```python
from build123d import *

# Parameters (mm, degrees)
BOLT_CIRCLE_R                                     = 14.2748
BOLT_CIRCLE_R_2                                   = 6.35
BASE_DEPTH                                        = 12.7
STRUCTURE_TUBE_CONNECTION_COUNTERBORE_D           = 6.7564
STRUCTURE_TUBE_CONNECTION_COUNTERBORE_CBORE_D     = 11.1125
STRUCTURE_TUBE_CONNECTION_COUNTERBORE_CBORE_DEPTH = 6.35
STRUCTURE_TUBE_CONNECTION_COUNTERBORE_PA_COUNT    = 4
SPINDLE_CONNECTION_COUNTERBORE_D                  = 6.7564
SPINDLE_CONNECTION_COUNTERBORE_CBORE_D            = 11.1125
SPINDLE_CONNECTION_COUNTERBORE_CBORE_DEPTH        = 6.35
SPINDLE_CONNECTION_COUNTERBORE_PATTERN_COUNT      = 4
SKETCH16_R                                        = 36.5125
STRUCTURE_TUBE_MOUNTING_POCKET_DEPTH              = 6.35
SKETCH17_R                                        = 36.5125
SPINDLE_MOUNTING_POCKET_DEPTH                     = 7.62
SKETCH18_R                                        = 9.525
LEAD_SCREW_THROUGH_HOLE_DEPTH                     = 9.525
SKETCH20_R                                        = 7.9375
RAIL_MOUNTING_PILOT_HOLES_DEPTH                   = 166.290695159
SKETCH27_R                                        = 2.38125
ALIGNMENT_FEATURES_DEPTH                          = 6.35
GENERIC_ROUNDING_FILLET_R                         = 6.35
WOOD_SPINDLE_CBORE_D                              = 6.7564
WOOD_SPINDLE_CBORE_CBORE_D                        = 11.1125
WOOD_SPINDLE_CBORE_CBORE_DEPTH                    = 6.35
CIRPATTERN1_COUNT                                 = 4
SKETCH30_R                                        = 36.5125
CUT_EXTRUDE1_DEPTH                                = 7.62


with BuildPart() as part:
    # Bolt circle → Base (new, symmetric)
    with BuildSketch(Plane.XY):
        with BuildLine():
            Line((-42.8625, 76.2), (-42.8625, -77.7875))
            Line((-42.8625, -77.7875), (-69.85, -77.7875))
            Line((-69.85, -77.7875), (-69.85, -147.6375))
            Line((-69.85, -147.6375), (69.85, -147.6375))
            Line((69.85, -147.6375), (69.85, -77.7875))
            Line((69.85, -77.7875), (42.8625, -77.7875))
            Line((42.8625, -77.7875), (42.8625, 76.2))
            ThreePointArc((42.8625, 76.2), (0, 119.0625), (-42.8625, 76.2))
        make_face()
        with Locations((0, 76.2)):
            Circle(BOLT_CIRCLE_R, mode=Mode.SUBTRACT)
        Circle(BOLT_CIRCLE_R, mode=Mode.SUBTRACT)
        with Locations((0, -98.425)):
            Circle(BOLT_CIRCLE_R_2, mode=Mode.SUBTRACT)
    extrude(amount=BASE_DEPTH, both=True)

    # Structure tube connection counterbore (through all)
    with Locations(Plane(origin=(0, 0, -12.7), x_dir=(-1, 0, 0), z_dir=(0, 0, -1))):
        with Locations((0, -67.46875)):
            structure_tube_connection_counterbore = CounterBoreHole(STRUCTURE_TUBE_CONNECTION_COUNTERBORE_D / 2, STRUCTURE_TUBE_CONNECTION_COUNTERBORE_CBORE_D / 2, STRUCTURE_TUBE_CONNECTION_COUNTERBORE_CBORE_DEPTH)

    # Structure tube connection counterbore pa: Structure tube connection counterbore ×4 about axis
    structure_tube_connection_counterbore_pa_axis = Axis((0, -98.425, 0), (0, 0, 1))
    for i in range(1, STRUCTURE_TUBE_CONNECTION_COUNTERBORE_PA_COUNT):
        add(structure_tube_connection_counterbore.rotate(structure_tube_connection_counterbore_pa_axis, i * 360 / STRUCTURE_TUBE_CONNECTION_COUNTERBORE_PA_COUNT), mode=Mode.SUBTRACT)

    # Spindle connection counterbore (through all)
    with Locations(Plane.XY.offset(12.7)):
        with Locations((0, 31.75)):
            spindle_connection_counterbore = CounterBoreHole(SPINDLE_CONNECTION_COUNTERBORE_D / 2, SPINDLE_CONNECTION_COUNTERBORE_CBORE_D / 2, SPINDLE_CONNECTION_COUNTERBORE_CBORE_DEPTH)

    # Spindle connection counterbore pattern: Spindle connection counterbore ×4 about axis
    spindle_connection_counterbore_pattern_axis = Axis((0, 0, 0), (0, 0, 1))
    for i in range(1, SPINDLE_CONNECTION_COUNTERBORE_PATTERN_COUNT):
        add(spindle_connection_counterbore.rotate(spindle_connection_counterbore_pattern_axis, i * 360 / SPINDLE_CONNECTION_COUNTERBORE_PATTERN_COUNT), mode=Mode.SUBTRACT)

    # Sketch16 → Structure tube mounting pocket (cut)
    with BuildSketch(Plane.XY.offset(12.7)):
        with Locations((0, -98.425)):
            Circle(SKETCH16_R)
    extrude(amount=-STRUCTURE_TUBE_MOUNTING_POCKET_DEPTH, mode=Mode.SUBTRACT)

    # Sketch17 → Spindle mounting pocket (cut)
    with BuildSketch(Plane(origin=(0, 0, -12.7), x_dir=(-1, 0, 0), z_dir=(0, 0, -1))):
        Circle(SKETCH17_R)
    extrude(amount=-SPINDLE_MOUNTING_POCKET_DEPTH, mode=Mode.SUBTRACT)

    # Sketch18 → Lead screw through hole (cut)
    with BuildSketch(Plane.XY.offset(6.35)):
        with Locations((0, -98.425)):
            Circle(SKETCH18_R)
    extrude(amount=-LEAD_SCREW_THROUGH_HOLE_DEPTH, mode=Mode.SUBTRACT)

    # Sketch20 → Rail mounting pilot_holes (cut, through all)
    with BuildSketch(Plane.XY.offset(12.7)):
        with Locations((57.15, -98.425)):
            Circle(SKETCH20_R)
        with Locations((-57.15, -98.425)):
            Circle(SKETCH20_R)
    extrude(amount=-RAIL_MOUNTING_PILOT_HOLES_DEPTH, mode=Mode.SUBTRACT)

    # Sketch27 → Alignment_features (cut)
    with BuildSketch(Plane.XY.offset(6.35)):
        with Locations((-21.889374295, -120.314374295)):
            Circle(SKETCH27_R)
        with BuildLine():
            Line((20.681324246, -74.335397148), (19.602797121, -75.500272889))
            ThreePointArc((19.602797121, -75.500272889), (19.732320046, -78.865377187), (23.097424344, -78.735854262))
            Line((23.097424344, -78.735854262), (24.175951469, -77.570978521))
            ThreePointArc((24.175951469, -77.570978521), (24.046428544, -74.205874223), (20.681324246, -74.335397148))
        make_face()
    extrude(amount=-ALIGNMENT_FEATURES_DEPTH, mode=Mode.SUBTRACT)

    # Generic_rounding_fillet
    generic_rounding_fillet_edges = [part.edges().sort_by_distance(p)[0] for p in [
        (-42.8625, -77.7875, 0),
        (42.8625, -77.7875, 0),
        (69.85, -147.6375, 0),
        (-69.85, -147.6375, 0),
    ]]
    fillet(generic_rounding_fillet_edges, radius=GENERIC_ROUNDING_FILLET_R)

    # wood_spindle_CBORE (through all)
    with Locations(Plane.XY.offset(12.7)):
        with Locations((0, 107.15625)):
            wood_spindle_cbore = CounterBoreHole(WOOD_SPINDLE_CBORE_D / 2, WOOD_SPINDLE_CBORE_CBORE_D / 2, WOOD_SPINDLE_CBORE_CBORE_DEPTH)

    # CirPattern1: wood_spindle_CBORE ×4 about axis
    cirpattern1_axis = Axis((0, 76.2, 0), (0, 0, 1))
    for i in range(1, CIRPATTERN1_COUNT):
        add(wood_spindle_cbore.rotate(cirpattern1_axis, i * 360 / CIRPATTERN1_COUNT), mode=Mode.SUBTRACT)

    # Sketch30 → Cut-Extrude1 (cut)
    with BuildSketch(Plane(origin=(0, 0, -12.7), x_dir=(-1, 0, 0), z_dir=(0, 0, -1))):
        with Locations((0, 76.2)):
            Circle(SKETCH30_R)
    extrude(amount=-CUT_EXTRUDE1_DEPTH, mode=Mode.SUBTRACT)


solid = part.part
```
Source: CAD feature listing. Evaluate the final solid. Frame: model axes, mm. A direction names the side the tool comes from. Give positions to 0.01 mm unless a question says otherwise; leave off trailing zeros. Write each loop counter-clockwise with the first axis right and the second up, starting at its lowest first coordinate (ties: lowest second). Pieces come first, ordered by that corner, then holes.
1. Section query D-D (y = -31.75). Return the cut outline in (x, z).
2. Material intervals for line 1 along Y through (x, z) = (0, -10.25) (1 decimal); line 2 along Y through (x, z) = (29.5, 3); line 3 along Y through (x, z) = (-4.5, -5.5), sorted ascending.
3. First-contact query: pin 1 (12 mm diameter, centred on x = 23.5, z = 5.5, fed in from +Y); pin 2 (4 mm diameter, centred on x = -21.89, y = -120.31, fed in from +Z); pin 3 (3.5 mm diameter, centred on x = -2, y = -30, fed in from +Z). Flat tips, straight axial feed; report the tip coordinate or a pass-through.
4. Pull-direction query (Y, two-part tool) for faces 4 (the face through (-42.862, 3, 0)), 5 (the face through (60, -77.788, 0)), 6 (the face through (-1.377, -104.624, -8.004)), 7 (the face through (-0.73, -28.45, 0.55)); classes: +Y half, -Y half, draft (parallel to the pull), parting line (faces both ways), or undercut.
5. Section query A-A (y = 0). Return the cut outline in (x, z).
6. Access query for faces 1 (the face through (-0.72, -134.89, -9.57)), 2 (the face through (-22, -120, 0)), 3 (the face through (15, -12, 12.7)). Directions: +Z, -Z, +X, -X, +Y, -Y. A direction counts if a zero-diameter tool reaches every point of the face in a straight line with its end or side. Return the directions, or none.
7. Section query B-B (x = -57.15). Return the cut outline in (y, z).
8. Section query C-C (z = 9.5). Count the separate pieces of the cut face and the enclosed holes in it, then the cut area to 3 significant figures.
Output values:
1. outline: (-42.86, -12.7) - (-18.03, -12.7) - (-18.03, -5.08) - (-3.38, -5.08) - (-3.38, 6.35) - (-5.56, 6.35) - (-5.56, 12.7) - (-42.86, 12.7) - close; (3.38, -5.08) - (18.03, -5.08) - (18.03, -12.7) - (42.86, -12.7) - (42.86, 12.7) - (5.56, 12.7) - (5.56, 6.35) - (3.38, 6.35) - close
2. line 1: y = -147.6 to -134.9, -123.8 to -104.8, -92.1 to -73, -61.9 to -36.5, 36.5 to 39.7, 112.7 to 119.1
2. line 2: y = -147.64 to -101.47, -95.38 to -2.52, 2.52 to 73.15, 79.25 to 107.3
2. line 3: y = -147.64 to -102.91, -93.94 to -36.23, 36.23 to 39.97, 112.43 to 118.83
3. pin 1: stops at y = 115.33
3. pin 2: stops at z = 0
3. pin 3: stops at z = 6.35
4. face 4: draft
4. face 5: +Y half
4. face 6: undercut
4. face 7: undercut
5. outline: (-42.86, -12.7) - (-36.51, -12.7) - (-36.51, -5.08) - (-35.13, -5.08) - (-35.13, 6.35) - (-37.31, 6.35) - (-37.31, 12.7) - (-42.86, 12.7) - close; (-28.37, -5.08) - (-14.27, -5.08) - (-14.27, 12.7) - (-26.19, 12.7) - (-26.19, 6.35) - (-28.37, 6.35) - close; (14.27, -5.08) - (28.37, -5.08) - (28.37, 6.35) - (26.19, 6.35) - (26.19, 12.7) - (14.27, 12.7) - close; (35.13, -5.08) - (36.51, -5.08) - (36.51, -12.7) - (42.86, -12.7) - (42.86, 12.7) - (37.31, 12.7) - (37.31, 6.35) - (35.13, 6.35) - close
6. face 1: -Z
6. face 2: +Z
6. face 3: +Z, +X, -X, +Y, -Y
7. outline: (-147.64, -12.7) - (-106.36, -12.7) - (-106.36, 12.7) - (-147.64, 12.7) - close; (-90.49, -12.7) - (-77.79, -12.7) - (-77.79, 12.7) - (-90.49, 12.7) - close
8. separate pieces: 1
8. enclosed holes: 13
8. area: 19,200 mm2
